Work out the finished part from the listing and answer in its coordinate system (mm). Face numbers are marked on the shaded views. Coordinates: 2 decimals unless noted, no trailing zeros. Order: outer loops, then holes, each group sorted by start corner. A loop starts at its lowest first (then second) coordinate and runs counter-clockwise, first axis right, second up. Notation, with made-up numbers: M 46.5,30.25 L 89.5,30.25 A32 cw 89.5,56.25 Z; hole C 2,-8.5 d5. An arc over 180 degrees is marked long. Use a Markdown table: item, result.
from build123d import *

# Parameters (mm, degrees)
F0_R     = 43.18
F1_DEPTH = 76.2
F3_DEPTH = 76.201
F4_R     = 38.1
F5_DEPTH = 67.31
F6_W     = 3.81
F6_H     = 2.54


with BuildPart() as f1:
    # F0 (on Front) → F1 (new body)
    with BuildSketch(Plane.XZ):
        Circle(F0_R)
    extrude(amount=-F1_DEPTH)

    # F2 (on Front) → F3 (cut, through all)
    with BuildSketch(Plane.XZ):
        Polygon((-21.434986513, 25.8488521843), (-35.4417645981, -12.2166163401), (-31.9433667717, -12.2166163401), (-17.9365886866, 25.8488521843), align=None)
        Polygon((-22.0389613365, -12.2166163401), (-10.2934986338, -12.2166163401), (3.7132794513, 25.8488521843), (-8.0321832514, 25.8488521843), align=None)
        Polygon((-16.8483592018, 25.8488521843), (-30.8551372869, -12.2166163401), (-23.1931219477, -12.2166163401), (-9.1863438626, 25.8488521843), align=None)
        with BuildLine():
            Line((4.7790936304, 25.8488521843), (0.4074209647, 13.9681921752))
            Line((0.4074209647, 13.9681921752), (13.1397311344, 13.9681921752))
            add(Edge.make_bspline(
                [(13.1397311344, 13.9681921752), (13.5623199674, 13.4908529986), (14.4433645606, 12.4956608219), (14.2607531046, 10.2552541119), (13.2775679328, 7.9123953601), (12.6805237168, 7.4737343771), (12.4528049578, 7.3064246)],
                knots=[0, 0, 0, 0, 0.2524611124, 0.5263496824, 0.8193449335, 1, 1, 1, 1], degree=3))
            Line((12.4528049578, 7.3064246), (-1.9049127084, 7.3064246))
            Line((-1.9049127084, 7.3064246), (-6.6714608383, -5.6473672505))
            Line((-6.6714608383, -5.6473672505), (3.8388244906, -24.9511478157))
            Line((3.8388244906, -24.9511478157), (20.2734413777, -24.9511478157))
            Line((20.2734413777, -24.9511478157), (24.1563424543, -12.1285331834))
            Line((24.1563424543, -12.1285331834), (14.6748356249, -12.1285331834))
            Line((14.6748356249, -12.1285331834), (10.0151892599, -3.5703648629))
            Line((10.0151892599, -3.5703648629), (20.99584212, -3.5703648629))
            add(Edge.make_bspline(
                [(23.8076338339, 25.8488521843), (24.8241026662, 25.3389018018), (26.9075174339, 24.2936772717), (29.0501970552, 21.1204133476), (30.72383942, 15.9362694954), (30.1770180196, 10.5156157051), (28.7431916568, 4.5225535349), (25.4079508495, -0.3677177865), (22.4492557888, -2.5153656953), (20.99584212, -3.5703648629)],
                knots=[0, 0, 0, 0, 0.1175129286, 0.2408614638, 0.3885970952, 0.5383784175, 0.6968239202, 0.8510693906, 1, 1, 1, 1], degree=3))
            Line((23.8076338339, 25.8488521843), (4.7790936304, 25.8488521843))
        make_face()
    extrude(amount=-F3_DEPTH, mode=Mode.SUBTRACT)

    # F4 (on face) → F5 (cut)
    with BuildSketch(Plane(origin=(0, 76.2, 0), x_dir=(-1, 0, 0), z_dir=(0, 1, 0))):
        Circle(F4_R)
    extrude(amount=-F5_DEPTH, mode=Mode.SUBTRACT)

    # F6 (on Right) → F7 (revolve, cut)
    with BuildSketch(Plane.YZ):
        with Locations((6.985, 42.0579532842)):
            Rectangle(F6_W, F6_H)
        with Locations((18.415, 42.0579532842)):
            Rectangle(F6_W, F6_H)
    revolve(axis=Axis((0, 34.9276592024, 0), (0, -1, 0)), mode=Mode.SUBTRACT)


solid = f1.part
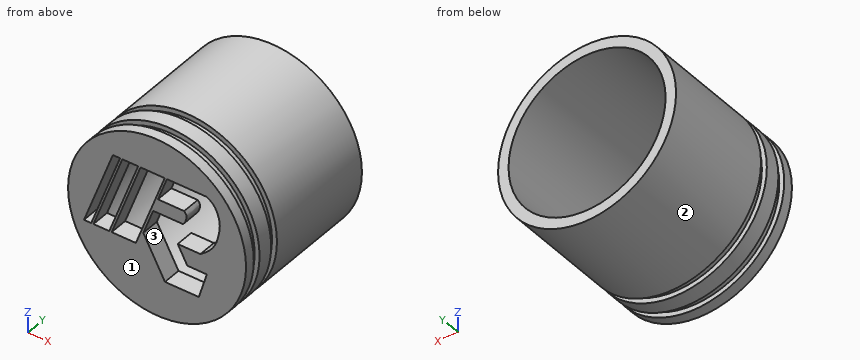
1. Flat-ended cylindrical pins translate along their axes: P1, Ø4.5, axis at x = -17.5, y = 4, coming from the +Z side; P2, Ø4, axis at x = -29, y = 3.5, coming from the +Z side; P3, Ø7, axis at x = 6, y = 3, coming from the -Z side. Find the tip coordinate at first contact, or state that the pin passes through.
Answers below:
| item | result |
|---|---|
| P1 | z = 40.4 |
| P2 | z = 33.7 |
| P3 | z = -43.11 |
2. Find the intervals of material crossed by probe 1 along Y at (x, z) = (37, 20.5); probe 2 along X at (y, z) = (6.5, 2); probe 3 along X at (y, z) = (6.5, 10.5), in increasing order.
Answers below:
| item | result |
|---|---|
| probe 1 | 0 to 5.08, 8.89 to 16.51, 20.32 to 76.2 |
| probe 2 | -40.74 to -30.21, -26.71 to -25.62, -17.96 to -16.81, -5.06 to -3.86, 26.92 to 40.74 |
| probe 3 | -39.41 to -27.08, -23.58 to -22.5, -14.83 to -13.68, -1.93 to 14.18, 30.04 to 39.41 |
3. Section C-C on y = 50.5 is taken. Determine the outline of the cut face in (x, z).
Answers below:
| item | result |
|---|---|
| outline | C 0,0 d86.36; hole C 0,0 d76.2 |
4. For a pull along Z with two mould halves and no side action, classify the marked faces 1, 2 and 3 as +Z half, -Z half, draft (parallel to the pull), parting line (faces both ways), or undercut.
Answers below:
| item | result |
|---|---|
| face 1 | draft |
| face 2 | parting line |
| face 3 | undercut |
5. Section B-B on z = -16.5 is taken. Determine the outline of the cut face in (x, y).
Answers below:
| item | result |
|---|---|
| outline | M -39.9,0 L -0.76,0 L -0.76,8.89 L -34.34,8.89 L -34.34,76.2 L -39.9,76.2 L -39.9,20.32 L -37.3,20.32 L -37.3,16.51 L -39.9,16.51 L -39.9,8.89 L -37.3,8.89 L -37.3,5.08 L -39.9,5.08 Z; M 22.83,0 L 39.9,0 L 39.9,5.08 L 37.3,5.08 L 37.3,8.89 L 39.9,8.89 L 39.9,16.51 L 37.3,16.51 L 37.3,20.32 L 39.9,20.32 L 39.9,76.2 L 34.34,76.2 L 34.34,8.89 L 22.83,8.89 Z |
6. Section D-D on z = 28 is taken. Determine the outline of the cut face in (x, y), then the cut area to 3 significant figures.
Answers below:
| item | result |
|---|---|
| outline | M -32.87,0 L 32.87,0 L 32.87,5.08 L 29.66,5.08 L 29.66,8.89 L 32.87,8.89 L 32.87,16.51 L 29.66,16.51 L 29.66,20.32 L 32.87,20.32 L 32.87,76.2 L 25.84,76.2 L 25.84,8.89 L -25.84,8.89 L -25.84,76.2 L -32.87,76.2 L -32.87,20.32 L -29.66,20.32 L -29.66,16.51 L -32.87,16.51 L -32.87,8.89 L -29.66,8.89 L -29.66,5.08 L -32.87,5.08 Z |
| area | 1,480 mm² |
7. Section A-A on x = -4 is taken. Give the number of separate pieces and of enclosed holes in the cut face, then the cut area to 3 significant figures.
Answers below:
| item | result |
|---|---|
| separate pieces | 3 |
| enclosed holes | 0 |
| area | 1,120 mm² |
